Autodesk Inventor part; units mm, degrees
ref_plane "YZ Plane" through (0, 0, 0) normal (1, 0, 0) x (0, 1, 0)
ref_plane "XZ Plane" through (0, 0, 0) normal (0, 1, 0) x (-1, 0, 0)
ref_plane "XY Plane" through (0, 0, 0) normal (0, 0, 1) x (1, 0, 0)
sketch "Sketch1" plane through (0, 0, 0) normal (1, 0, 0) x (0, 1, 0)
  line L0 (-10.9728, 10.9728) -> (10.9728, 10.9728)
  line L1 (10.9728, 10.9728) -> (10.9728, -10.9728)
  line L2 (10.9728, -10.9728) -> (-10.9728, -10.9728)
  line L3 (-10.9728, -10.9728) -> (-10.9728, 10.9728)
  line L4 (-10.9728, 10.9728) -> (10.9728, -10.9728) construction
  line L5 (10.9728, 10.9728) -> (-10.9728, -10.9728) construction
  line L6 (-12.7, 12.7) -> (12.7, 12.7)
  line L7 (12.7, 12.7) -> (12.7, -12.7)
  line L8 (12.7, -12.7) -> (-12.7, -12.7)
  line L9 (-12.7, -12.7) -> (-12.7, 12.7)
  line L10 (-12.7, 12.7) -> (12.7, -12.7) construction
  line L11 (12.7, 12.7) -> (-12.7, -12.7) construction
  point P0 (0, 0)
  dimension "d2" = 1.7272
  dimension "d4" = 1.7272
  dimension "d5" = 25.4
  dimension "d6" = 25.4
extrude "Extrusion1" add sketch "Sketch1" along normal blind 381
sketch "Sketch2" plane through (0, -12.7, 12.7) normal (0, 0, 1) x (1, 0, 0)
  line L0 (0, 0) -> (0, 25.4)
  line L1 (381, 25.4) -> (381, 0)
  line L2 (0, 25.4) -> (381, 25.4)
  point P0 (0, 12.7)
  point P1 (25.4, 12.7)
  point P2 (355.6, 12.7)
  dimension "d9" = 25.4
  dimension "d10" = 12.7
  dimension "d11" = 25.4
  dimension "d12" = 12.7
hole "Hole1" at (25.4, 0, 12.7) at (355.6, 0, 12.7) direction (0, 0, -1) diameter 6.35 end through all
sketch "Sketch3" plane through (0, -12.7, 12.7) normal (0, 0, 1) x (1, 0, 0)
  line L0 (0, 0) -> (381, 0)
  line L1 (381, 25.4) -> (381, 0)
  line L2 (0, 25.4) -> (381, 25.4)
  line L3 (101.6, 25.4) -> (101.6, 0)
  line L4 (279.4, 25.4) -> (279.4, 0)
  line L5 (190.5, 25.4) -> (190.5, 0)
  point P0 (0, 12.7)
  point P1 (76.2, 12.7)
  point P2 (127, 12.7)
  point P3 (511.7916, 13.2861)
  point P4 (652.1971, 7.6456)
  point P5 (254, 12.7)
  point P6 (304.8, 12.7)
  dimension "d20" = 50.8
  dimension "d22" = 12.7
  dimension "d23" = 12.7
  dimension "d24" = 50.8
  dimension "d25" = 12.7
  dimension "d26" = 12.7
  dimension "d27" = 25.4
  dimension "d28" = 25.4
  dimension "d29" = 177.8
  dimension "d30" = 88.9
  dimension "d31" = 381
  dimension "d32" = 190.5
hole "Hole2" at (76.2, 0, 12.7) at (127, 0, 12.7) at (511.7916, 0.5861, 12.7) at (652.1971, -5.0544, 12.7) at (254, 0, 12.7) at (304.8, 0, 12.7) direction (0, 0, -1) diameter 6.35 end through all
sketch "Sketch4" plane through (0, 12.7, 12.7) normal (0, 1, 0) x (1, 0, 0)
  line L0 (381, 25.4) -> (381, 0)
  line L1 (0, 25.4) -> (381, 25.4)
  point P0 (0, 12.7)
  point P1 (190.5, 12.7)
  dimension "d40" = 12.7
  dimension "d41" = 190.5
hole "Hole3" at (190.5, 12.7, 0) direction (0, -1, 0) diameter 6.35 end through all
properties part number "BackBottonSupport" material "Aluminum 6061"
Model file for the job. Use its own axes, mm. A direction names the side the tool comes from. Round coordinates to 2 decimals unless told otherwise and drop trailing zeros. Write each loop counter-clockwise with the first axis right and the second up, starting at its lowest first coordinate (ties: lowest second). Pieces come first, ordered by that corner, then holes. Notation, with made-up numbers: (64.5, 27.25) -> (104.5, 27.25) arc R7 ccw to (104.5, 35.25) -> close; hole circle Ø11 at (82, 73). An arc over 180 degrees is marked (long way). Answer as CSV lines item,"result".
1. Slice it at A-A, the plane z = 0. List the corners of the cut face in (x, y) (3 decimals), plus the area to 3 significant figures.
Resolved:
outline,"(0, -12.7) -> (187.325, -12.7) -> (187.325, -10.973) -> (0, -10.973) -> close; (0, 10.973) -> (187.325, 10.973) -> (187.325, 12.7) -> (0, 12.7) -> close; (193.675, -12.7) -> (381, -12.7) -> (381, -10.973) -> (193.675, -10.973) -> close; (193.675, 10.973) -> (381, 10.973) -> (381, 12.7) -> (193.675, 12.7) -> close"
area,"1,290 mm²"
2. Drill centre lines: line 1 (Z direction, x = 210, y = 2.5); line 2 (Y direction, x = 254, z = 12.15) (3 decimals). Where is each one in solid material? Low to high.
Resolved:
line 1,"-12.7 to -10.97, 10.97 to 12.7"
line 2,"-12.7 to -3.175, 3.175 to 12.7"
3. Slice it at B-B, the plane x = 25.4. List the corners of the cut face in (y, z) (3 decimals).
Resolved:
outline,"(-12.7, -12.7) -> (-3.175, -12.7) -> (-3.175, -10.973) -> (-10.973, -10.973) -> (-10.973, 10.973) -> (-3.175, 10.973) -> (-3.175, 12.7) -> (-12.7, 12.7) -> close; (3.175, -12.7) -> (12.7, -12.7) -> (12.7, 12.7) -> (3.175, 12.7) -> (3.175, 10.973) -> (10.973, 10.973) -> (10.973, -10.973) -> (3.175, -10.973) -> close"
4. Pin check, flat tips, straight feed: pin 1 Ø10 at (x, y) = (127, 0) entering from -Z; pin 2 Ø5 at (x, z) = (190.5, 0) entering from +Y. Stop position of each tip, or through.
Resolved:
pin 1,"z = -12.7"
pin 2,"through"
5. Mould opens along X. For faces 1 (the face through (79.3, 0.69, 11.82)), 2 (the face through (381, -0.2, 11.5)), 3 (the face through (352.45, 0.41, -11.85)), 4 (the face through (188, 0, 12.7)) say: +X half, -X half, draft (parallel to the pull), parting line (faces both ways), or undercut.
Resolved:
face 1,"undercut"
face 2,"+X half"
face 3,"undercut"
face 4,"draft"
6. Slice it at C-C, the plane y = 0. State how many separate pieces and enclosed holes the cut face has, plus the area to 3 significant figures.
Resolved:
separate pieces,"14"
enclosed holes,"0"
area,"1,180 mm²"
7. Tool access for faces 5 (the face through (188, 0, -12.7)), 6 (the face through (188, 0, -10.973)): list every direction of +Z, -Z, +X, -X, +Y, -Y with a clear straight run to the whole face (end or side of a thin tool).
Resolved:
face 5,"-Z, +X, -X, +Y, -Y"
face 6,"+X, -X"
